Can you work these out from the drawing? Everything is in mm from the part's minimum corner. A direction names the side the tool comes from. Round coordinates to 2 decimals unless told otherwise and drop trailing zeros. Order: outer loops, then holes, each group sorted by start corner. A loop starts at its lowest first (then second) coordinate and runs counter-clockwise, first axis right, second up. Notation, with made-up numbers: (-39, -24) -> (6, -24) arc R32 ccw to (6, 3) -> close; hole circle Ø4 at (-36.75, -29.75). An arc over 180 degrees is marked (long way). Use a Markdown table: item, result. Add a question column.
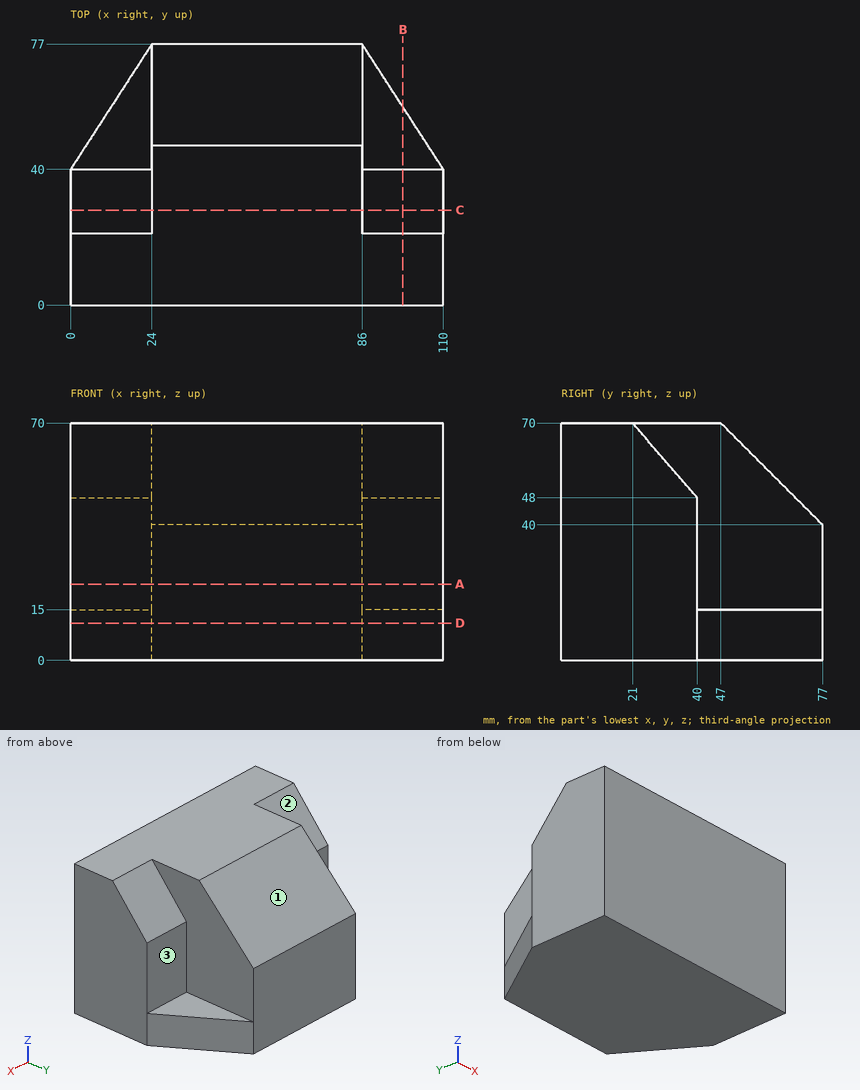
(1) I want a section at C-C on y = 28. List the corners of the cut face in (x, z) for me.
(2) Please list where these lines run through material, in increasing order: probe 1 along X at (y, z) = (63, 45); probe 2 along Y at (x, z) = (15, 30); probe 3 along Z at (x, y) = (15, 45). Write a range as from..to.
(3) I'm going to push flat-ended pins straight in: P1, Ø12, axis at x = 11.5, y = 53, coming from the +Z side; P2, Ø1.5, axis at x = 67, y = 69, coming from the +Z side; P3, Ø16.5, axis at y = 57.5, z = 40.5, coming from the -X side. Where does each tip first touch, or does it pass through?
(4) I want a section at B-B on x = 98. List the corners of the cut face in (y, z) for me, and give its area (3 significant figures).
(5) I want a section at D-D on z = 11. List the corners of the cut face in (x, y) for me.
(6) I want a section at A-A on z = 22.5. List the corners of the cut face in (x, y) for me.
(7) On a 3-axis mill with a long thin cutter (end or side, diameter ignored), from which of +Z, -Z, +X, -X, +Y, -Y can I reach the whole of each face in a straight line? I mean the marked faces 1, 2 and 3. Say none if no direction works.
Output:
| question | item | result |
|---|---|---|
| 1 | outline | (0, 0) -> (110, 0) -> (110, 61.89) -> (86, 61.89) -> (86, 70) -> (24, 70) -> (24, 61.89) -> (0, 61.89) -> close |
| 2 | probe 1 | 24..86 |
| 2 | probe 2 | 0..40 |
| 2 | probe 3 | 0..15 |
| 3 | P1 | z = 15 |
| 3 | P2 | z = 48.75 |
| 3 | P3 | x = 24 |
| 4 | outline | (0, 0) -> (58.5, 0) -> (58.5, 15) -> (40, 15) -> (40, 48) -> (21, 70) -> (0, 70) -> close |
| 4 | area | 2,870 mm² |
| 5 | outline | (0, 0) -> (110, 0) -> (110, 40) -> (86, 77) -> (24, 77) -> (0, 40) -> close |
| 6 | outline | (0, 0) -> (110, 0) -> (110, 40) -> (86, 40) -> (86, 77) -> (24, 77) -> (24, 40) -> (0, 40) -> close |
| 7 | face 1 | +Z, +X, -X, +Y |
| 7 | face 2 | +Z, -X, +Y |
| 7 | face 3 | +Z, +X, +Y |
